from build123d import *

# Parameters (mm, degrees)
SKETCH1_R                = 19
BOSS_EXTRUDE1_DEPTH      = 3.5
SKETCH2_R                = 30
SKETCH2_R_2              = 19
SKETCH2_R_3              = 2.8
BOSS_EXTRUDE2_DEPTH      = 8
BOSS_EXTRUDE3_DEPTH      = 2
BOSS_EXTRUDE3_DEPTH_BACK = 8
SKETCH4_R                = 2.9
SKETCH5_R                = 5
BOSS_EXTRUDE4_DEPTH      = 3
CUT_EXTRUDE1_START       = -10
SKETCH3_R                = 19
CUT_EXTRUDE1_DEPTH       = 10
SKETCH6_R                = 3
SKETCH6_R_2              = 2.9
CUT_EXTRUDE2_DEPTH       = 3
CUT_EXTRUDE3_START       = -13
CUT_EXTRUDE3_DEPTH       = 13
FILLET1_R                = 10
FILLET2_R                = 5


with BuildPart() as part:
    # Sketch1 → Boss-Extrude1 (new body)
    with BuildSketch(Plane(origin=(0, 0, 0), x_dir=(1, 0, 0), z_dir=(0, 1, 0))):
        with Locations(Location((0, 0, 0), (0, 0, 270))):
            Circle(SKETCH1_R)
    extrude(amount=BOSS_EXTRUDE1_DEPTH)

    # Sketch2 → Boss-Extrude2 (add)
    with BuildSketch(Plane(origin=(0, 0, 0), x_dir=(1, 0, 0), z_dir=(0, 1, 0))):
        with Locations(Location((0, 0, 0), (0, 0, 270))):
            Circle(SKETCH2_R)
        with Locations(Location((0, 0, 0), (0, 0, 270))):
            Circle(SKETCH2_R_2, mode=Mode.SUBTRACT)
        with Locations(Location((0, 25, 0), (0, 0, 270))):
            Circle(SKETCH2_R_3, mode=Mode.SUBTRACT)
        with Locations(Location((21.650635095, -12.5, 0), (0, 0, 270))):
            Circle(SKETCH2_R_3, mode=Mode.SUBTRACT)
        with Locations(Location((-21.650635095, -12.5, 0), (0, 0, 270))):
            Circle(SKETCH2_R_3, mode=Mode.SUBTRACT)
    extrude(amount=BOSS_EXTRUDE2_DEPTH)

    # Sketch4 → Boss-Extrude3 (add, two sides: drawn at the far end of the back side and taken through both)
    with BuildSketch(Plane.XZ.offset(-BOSS_EXTRUDE3_DEPTH_BACK)):
        with Locations(Location((-21.650635095, 12.5, 0), (0, 0, 270))):
            Circle(SKETCH4_R)
        with Locations(Location((21.650635095, 12.5, 0), (0, 0, 270))):
            Circle(SKETCH4_R)
        with Locations(Location((0, -25, 0), (0, 0, 270))):
            Circle(SKETCH4_R)
    extrude(amount=BOSS_EXTRUDE3_DEPTH + BOSS_EXTRUDE3_DEPTH_BACK)

    # Sketch5 → Boss-Extrude4 (add)
    with BuildSketch(Plane(origin=(0, 8, 0), x_dir=(1, 0, 0), z_dir=(0, 1, 0))):
        with Locations((-26.103110985, -14.7860609)):
            Circle(SKETCH5_R)
        with Locations((0.246451131, 29.99898768)):
            Circle(SKETCH5_R)
        with Locations((25.856659853, -15.212926781)):
            Circle(SKETCH5_R)
    extrude(amount=-BOSS_EXTRUDE4_DEPTH)

    # Sketch3 → Cut-Extrude1 (cut)
    with BuildSketch(Plane(origin=(0, 3.5, 0), x_dir=(1, 0, 0), z_dir=(0, 1, 0)).offset(CUT_EXTRUDE1_START)):
        with Locations(Location((0, 0, 0), (0, 0, 270))):
            Circle(SKETCH3_R)
    extrude(amount=CUT_EXTRUDE1_DEPTH, mode=Mode.SUBTRACT)

    # Sketch6 → Cut-Extrude2 (cut)
    with BuildSketch(Plane(origin=(0, 8, 0), x_dir=(1, 0, 0), z_dir=(0, 1, 0))):
        with Locations(Location((0, 25, 0), (0, 0, 270))):
            Circle(SKETCH6_R)
        with Locations(Location((21.650635095, -12.5, 0), (0, 0, 90))):
            Circle(SKETCH6_R_2)
        with Locations(Location((-21.650635095, -12.5, 0), (0, 0, 90))):
            Circle(SKETCH6_R_2)
    extrude(amount=-CUT_EXTRUDE2_DEPTH, mode=Mode.SUBTRACT)

    # Sketch7 → Cut-Extrude3 (cut)
    with BuildSketch(Plane(origin=(0, 8, 0), x_dir=(1, 0, 0), z_dir=(0, 1, 0)).offset(CUT_EXTRUDE3_START)):
        with BuildLine():
            ThreePointArc((-29.54423259, -5.20944533), (-25.980762114, 15), (-10.2606043, 28.190778624))
            Line((-10.2606043, 28.190778624), (-13.773984089, 37.84371026))
            Line((-13.773984089, 37.84371026), (-43.939319858, -7.747687605))
            Line((-43.939319858, -7.747687605), (-29.54423259, -5.20944533))
        make_face()
        with BuildLine():
            ThreePointArc((-21.729408673, -3.831481024), (-19.108521295, 11.032309914), (-7.546544436, 20.733960432))
            Line((-7.546544436, 20.733960432), (-10.2606043, 28.190778624))
            ThreePointArc((-10.2606043, 28.190778624), (-25.980762114, 15), (-29.54423259, -5.20944533))
            Line((-29.54423259, -5.20944533), (-21.729408673, -3.831481024))
        make_face()
        with BuildLine():
            Line((15.259965643, 41.926411025), (10.2606043, 28.190778624))
            ThreePointArc((10.2606043, 28.190778624), (25.980762114, 15), (29.54423259, -5.20944533))
            Line((29.54423259, -5.20944533), (39.660606503, -6.993234998))
            Line((39.660606503, -6.993234998), (15.259965643, 41.926411025))
        make_face()
        with BuildLine():
            Line((10.2606043, 28.190778624), (7.546544436, 20.733960432))
            ThreePointArc((7.546544436, 20.733960432), (18.074278438, 12.65574601), (22.064619828, 0))
            ThreePointArc((22.064619828, 0), (21.980657288, -1.92305833), (21.729408673, -3.831481024))
            Line((21.729408673, -3.831481024), (29.54423259, -5.20944533))
            ThreePointArc((29.54423259, -5.20944533), (25.980762114, 15), (10.2606043, 28.190778624))
        make_face()
        with BuildLine():
            Line((28.679354216, -34.17872342), (19.283628291, -22.981333294))
            ThreePointArc((19.283628291, -22.981333294), (0, -30), (-19.283628291, -22.981333294))
            Line((-19.283628291, -22.981333294), (-25.886622414, -30.850475262))
            Line((-25.886622414, -30.850475262), (28.679354216, -34.17872342))
        make_face()
        with BuildLine():
            Line((19.283628291, -22.981333294), (14.182864238, -16.902479408))
            ThreePointArc((14.182864238, -16.902479408), (0, -22.064619828), (-14.182864238, -16.902479408))
            Line((-14.182864238, -16.902479408), (-19.283628291, -22.981333294))
            ThreePointArc((-19.283628291, -22.981333294), (0, -30), (19.283628291, -22.981333294))
        make_face()
    extrude(amount=CUT_EXTRUDE3_DEPTH, mode=Mode.SUBTRACT)

    # Fillet1
    # the kernel refuses this fillet: 10 mm, written as the material it adds along each edge
    with BuildSketch(Plane(origin=(-21.729408673, 0, 3.831481024), x_dir=(-0.9848077530122133, 0, 0.17364817766690055), z_dir=(0, 1, 0)), Plane(origin=(14.182864238, 0, 16.902479408), x_dir=(0.6427876096865253, 0, 0.7660444431189899), z_dir=(0, 1, 0)), Plane(origin=(7.546544436, 0, -20.733960432), x_dir=(0.34202014332569675, 0, -0.9396926207858982), z_dir=(0, 1, 0))) as fillet1_piece_1:
        with BuildLine():
            CenterArc((8.404377584, -9.988996017), FILLET1_R, 92.688143309, 69.160575724)
            Line((-1.097995304, -6.873725644), (-1.288042762, -6.811420237))
            ThreePointArc((-1.288042762, -6.811420237), (-0.473724072, -3.448886874), (-0.2, 0))
            Line((-0.2, 0), (0, 0.2))
            ThreePointArc((0, 0.2), (3.967690086, 0.2), (7.926000224, 0.19977992))
            Line((7.926000224, 0.19977992), (7.935380172, 0))
        make_face()
    extrude(amount=8)
    with BuildSketch(Plane(origin=(-14.182864238, 0, 16.902479408), x_dir=(0.8578464941811706, 0, 0.5139060151633514), z_dir=(0, 1, 0)), Plane(origin=(21.729408673, 0, 3.831481024), x_dir=(0.016132417198510746, 0, -0.999869864089989), z_dir=(0, 1, 0)), Plane(origin=(-7.546544436, 0, -20.733960432), x_dir=(-0.8739789113796794, 0, 0.48596384892663586), z_dir=(0, 1, 0))) as fillet1_piece_2:
        with BuildLine():
            CenterArc((8.538251552, -9.87480959), FILLET1_R, 99.075640483, 69.160575724)
            Line((-1.251712984, -7.836036823), (-1.447512274, -7.795261367))
            ThreePointArc((-1.447512274, -7.795261367), (-0.823352684, -3.886470761), (-0.197496192, 0.03154765))
            Line((-0.197496192, 0.03154765), (0.03154765, 0.197496192))
            ThreePointArc((0.03154765, 0.197496192), (3.480434524, -0.07622788), (6.929321399, 0.197496192))
            Line((6.929321399, 0.197496192), (6.960869049, 0))
        make_face()
    extrude(amount=8)

    # Fillet2
    fillet2_edges = [part.edges().sort_by_distance(p)[0] for p in [
        (-19.283628291, 4, 22.981333294),
        (19.283628291, 4, 22.981333294),
        (29.54423259, 4, 5.20944533),
        (10.2606043, 4, -28.190778624),
        (-10.2606043, 4, -28.190778624),
        (-29.54423259, 4, 5.20944533),
    ]]
    fillet(fillet2_edges, radius=FILLET2_R)


solid = part.part
Could you check a few things on this model? Use its own coordinates, in mm. A direction names the side the tool comes from. Give positions to 0.01 mm unless a question says otherwise; leave off trailing zeros. Loops run counter-clockwise (first coordinate to the right, second up) from the corner with the lowest first, then second, coordinate; pieces in that order, holes last. Notation, with made-up numbers: (-33.75, 45) -> (13.25, 45) arc R32 cw to (13.25, 79) -> close; hole circle Ø1 at (-29.75, 87). An arc over 180 degrees is marked (long way). Return JSON: item names as keys, results as strings.
Item 1: If we section it at C-C on y = 6.5: Count the separate pieces of the cut face and the enclosed holes in it, plus the area to 3 significant figures.
Geometry results:
{"separate pieces": "1", "enclosed holes": "4", "area": "923 mm²"}
Item 2: I'm going to push flat-ended pins straight in: pin 1 (6 mm diameter, centred on y = 5, z = 4, fed in from +X); pin 2 (1.7 mm diameter, centred on x = 22.5, z = 12.5, fed in from +Y); pin 3 (2 mm diameter, centred on y = 7, z = -27, fed in from +X); pin 4 (8 mm diameter, centred on x = -4.5, z = -13.5, fed in from +Y). Where does each tip first touch, or does it pass through?
Geometry results:
{"pin 1": "stops at x = 28.54", "pin 2": "stops at y = 5", "pin 3": "stops at x = 9.6", "pin 4": "passes through"}
Item 3: If we section it at B-B on x = 0: List the corners of the cut face in (y, z) for me, plus the area to 3 significant figures.
Geometry results:
{"outline": "(-2, -27.9) -> (0, -27.9) -> (0, -30) -> (5, -30) -> (5, -34.99) -> (8, -34.99) -> (8, -28) -> (5, -28) -> (5, -22) -> (8, -22) -> (8, -19) -> (0, -19) -> (0, -22.1) -> (-2, -22.1) -> close; (0, 19) -> (8, 19) -> (8, 22.06) -> (0, 22.06) -> close", "area": "121 mm²"}
Item 4: I need wall thicknesses on L1, parallel to X at y = 6.95, z = 12.5; L2, parallel to X at y = 4, z = -16.5; L3, parallel to X at y = 3, z = -5.5. Which ranges of each line are inside material? Lowest first, please. Write a range as from..to.
Geometry results:
{"L1": "x = -30.55..-24.55, -18.75..-14.31, 14.31..18.75, 24.55..30.06", "L2": "x = -14.65..-9.42, 9.42..14.65", "L3": "x = -21.37..-18.19, 18.19..21.37"}
Item 5: We'd pull the mould along Z, two halves only. Please class faces 4 (the cylindrical face through (12.476, 3.944, 19.776)), 5 (the cylindrical face through (0.1, -1, -22.1)), 6 (the flat face through (-22, -2, 13)), 7 (the cylindrical face through (-21.778, 6.521, 15.397)): +Z half, -Z half, draft (parallel to the pull), parting line (faces both ways), or undercut.
Geometry results:
{"face 4": "+Z half", "face 5": "parting line", "face 6": "draft", "face 7": "undercut"}
Item 6: If we section it at D-D on z = -24: List the corners of the cut face in (x, y) for me, plus the area to 3 significant figures.
Geometry results:
{"outline": "(-9.88, 0) -> (-2.72, 0) -> (-2.72, -2) -> (2.72, -2) -> (2.72, 0) -> (9.88, 0) -> (9.88, 8) -> (2.83, 8) -> (2.83, 5) -> (-2.83, 5) -> (-2.83, 8) -> (-9.88, 8) -> close", "area": "152 mm²"}
Item 7: If we section it at A-A on z = -6: List the corners of the cut face in (x, y) for me, plus the area to 3 significant figures.
Geometry results:
{"outline": "(-21.23, 0) -> (-18.03, 0) -> (-18.03, 8) -> (-21.23, 8) -> close; (18.03, 0) -> (21.23, 0) -> (21.23, 8) -> (18.03, 8) -> close", "area": "51.3 mm²"}
Item 8: Which directions (+Z, -Z, +X, -X, +Y, -Y) give clear straight access to the entire face, cutting with the end or side of a thin tool? Please do faces 1 (the flat face through (22, -2, 13)), 2 (the flat face through (-13, 0, 15)), 3 (the flat face through (0, 5, -25)).
Geometry results:
{"face 1": "+Z, -Z, +X, -X, -Y", "face 2": "-Y", "face 3": "+Y"}
